The listing builds one solid part. Answer for the finished solid, in the listing's coordinates (mm). A direction names the side the tool comes from. Coordinates: 2 decimals unless noted, no trailing zeros. Order: outer loops, then holes, each group sorted by start corner. A loop starts at its lowest first (then second) coordinate and runs counter-clockwise, first axis right, second up. Notation, with made-up numbers: (-16.75, 38) -> (35.25, 38) arc R20 ccw to (35.25, 65) -> close; hole circle Ø11 at (75, 47). An arc over 180 degrees is marked (long way). Return JSON: item names as keys, results as strings.
```python
from build123d import *

# Parameters (mm, degrees)
SKETCH_2_W                = 80
SKETCH_2_H                = 104
SKETCH_2_R                = 2.25
EXTRUDE_1_DEPTH           = 7
HOLE_WIZARD_1_D           = 4.5
HOLE_WIZARD_1_CBORE_D     = 7.3
HOLE_WIZARD_1_CBORE_DEPTH = 4.2
CUT_EXTRUDE_1_DEPTH       = 2.5


with BuildPart() as part:
    # 草圖2 → 填料-伸長1 (new body)
    with BuildSketch(Plane.XY):
        Rectangle(SKETCH_2_W, SKETCH_2_H)
        with Locations((-18, 18)):
            Circle(SKETCH_2_R, mode=Mode.SUBTRACT)
        with Locations((-32.5, 47)):
            Circle(SKETCH_2_R, mode=Mode.SUBTRACT)
        with Locations((18, 18)):
            Circle(SKETCH_2_R, mode=Mode.SUBTRACT)
        with Locations((18, -18)):
            Circle(SKETCH_2_R, mode=Mode.SUBTRACT)
        with Locations((-18, -18)):
            Circle(SKETCH_2_R, mode=Mode.SUBTRACT)
        with Locations((32.5, 47)):
            Circle(SKETCH_2_R, mode=Mode.SUBTRACT)
        with Locations((32.5, -47)):
            Circle(SKETCH_2_R, mode=Mode.SUBTRACT)
        with Locations((-32.5, -47)):
            Circle(SKETCH_2_R, mode=Mode.SUBTRACT)
    extrude(amount=EXTRUDE_1_DEPTH)

    # 鑽孔1 (through all)
    with Locations(Plane(origin=(-18, 18, 7), x_dir=(1, 0, 0), z_dir=(0, 0, 1))):
        with Locations((0, 0), (36, 0), (36, -36), (0, -36)):
            CounterBoreHole(HOLE_WIZARD_1_D / 2, HOLE_WIZARD_1_CBORE_D / 2, HOLE_WIZARD_1_CBORE_DEPTH)

    # 草圖4 → 除料-伸長1 (cut)
    with BuildSketch(Plane(origin=(0, 0, 0), x_dir=(-1, 0, 0), z_dir=(0, 0, -1))):
        Polygon((-28.285343035, 47), (-30.392671517, 50.65), (-34.607328483, 50.65), (-36.714656965, 47), (-34.607328483, 43.35), (-30.392671517, 43.35), align=None)
        Polygon((30.392671517, 43.35), (28.285343035, 47), (30.392671517, 50.65), (34.607328483, 50.65), (36.714656965, 47), (34.607328483, 43.35), align=None)
        Polygon((28.285343035, -47), (30.392671517, -50.65), (34.607328483, -50.65), (36.714656965, -47), (34.607328483, -43.35), (30.392671517, -43.35), align=None)
        Polygon((-30.392671517, -43.35), (-28.285343035, -47), (-30.392671517, -50.65), (-34.607328483, -50.65), (-36.714656965, -47), (-34.607328483, -43.35), align=None)
    extrude(amount=-CUT_EXTRUDE_1_DEPTH, mode=Mode.SUBTRACT)


solid = part.part
```
Item 1: The part is cut by section B-B on y = 18. Determine the outline of the cut face in (x, z).
Answer list:
{"outline": "(-40, 0) -> (-20.25, 0) -> (-20.25, 2.8) -> (-21.65, 2.8) -> (-21.65, 7) -> (-40, 7) -> close; (-15.75, 0) -> (15.75, 0) -> (15.75, 2.8) -> (14.35, 2.8) -> (14.35, 7) -> (-14.35, 7) -> (-14.35, 2.8) -> (-15.75, 2.8) -> close; (20.25, 0) -> (40, 0) -> (40, 7) -> (21.65, 7) -> (21.65, 2.8) -> (20.25, 2.8) -> close"}
Item 2: The part is cut by section A-A on x = 32.5. Determine the outline of the cut face in (y, z), plus the area to 3 significant figures.
Answer list:
{"outline": "(-52, 0) -> (-50.65, 0) -> (-50.65, 2.5) -> (-49.25, 2.5) -> (-49.25, 7) -> (-52, 7) -> close; (-44.75, 2.5) -> (-43.35, 2.5) -> (-43.35, 0) -> (43.35, 0) -> (43.35, 2.5) -> (44.75, 2.5) -> (44.75, 7) -> (-44.75, 7) -> close; (49.25, 2.5) -> (50.65, 2.5) -> (50.65, 0) -> (52, 0) -> (52, 7) -> (49.25, 7) -> close", "area": "651 mm2"}
Item 3: Find the intervals of material crossed by probe 1 along Y at (x, z) = (18, 5.9); probe 2 along Y at (x, z) = (18, 1); probe 3 along X at (y, z) = (-16, 6), in increasing order.
Answer list:
{"probe 1": "-52 to -21.65, -14.35 to 14.35, 21.65 to 52", "probe 2": "-52 to -20.25, -15.75 to 15.75, 20.25 to 52", "probe 3": "-40 to -21.05, -14.95 to 14.95, 21.05 to 40"}
Item 4: Which of the six approach directions +Z, -Z, +X, -X, +Y, -Y give full straight-line access (tool end or side, diameter ignored) to faces 1 (the cylindrical face through (-16.962, 16.004, 1.38)), 2 (the flat face through (16, 16, 2.8)), 3 (the flat face through (-32, 50.65, 1))?
Answer list:
{"face 1": "+Z, -Z", "face 2": "+Z", "face 3": "-Z"}
Item 5: The part is cut by section C-C on z = 5.25. Count the separate pieces of the cut face and the enclosed holes in it, plus the area to 3 significant figures.
Answer list:
{"separate pieces": "1", "enclosed holes": "8", "area": "8,090 mm2"}
Item 6: Determine the mould class of faces 4 (the flat face through (-1, -52, 3)), 5 (the cylindrical face through (-31.29, -45.103, 4.719)), 6 (the flat face through (29.354, 45.149, 1.232)), 7 (the flat face through (-1, 52, 3)) for opening direction Y: pulls with the +Y half, pulls with the -Y half, needs draft (parallel to the pull), parting line crosses it, or undercut.
Answer list:
{"face 4": "pulls with the -Y half", "face 5": "undercut", "face 6": "undercut", "face 7": "pulls with the +Y half"}
Item 7: Flat-ended cylindrical pins translate along their axes: pin 1 (8.5 mm diameter, centred on x = 18, y = 18, fed in from +Z); pin 2 (4 mm diameter, centred on x = -18, y = -18, fed in from +Z); pin 3 (7 mm diameter, centred on x = 32.5, y = -47, fed in from -Z); pin 4 (6 mm diameter, centred on x = -18, y = 18, fed in from +Z). Find the tip coordinate at first contact, or state that the pin passes through.
Answer list:
{"pin 1": "z = 7", "pin 2": "through", "pin 3": "z = 2.5", "pin 4": "z = 2.8"}
